For this review, take the finished solid that the model builds, in its own axes (mm). A direction names the side the tool comes from. Round coordinates to 2 decimals unless told otherwise and drop trailing zeros. Loops run counter-clockwise (first coordinate to the right, second up) from the corner with the lowest first, then second, coordinate; pieces in that order, holes last.
1. Clearance check with flat-ended pins moving along their axes: pin 1 Ø3 at (x, z) = (-18.25, 14) entering from -Y; pin 2 Ø1.2 at (x, y) = (-29.25, -8) entering from +Z. State where each tip first meets the part, or that it passes through.
2. Consider section C-C on z = 3. State the section outline as (x, y) points, then the cut area to 3 significant figures.
3. To check wall thickness, follow line 1 along Y through (x, z) = (29.25, -8); line 2 along Y through (x, z) = (-30, 1.5); line 3 along X through (y, z) = (-31.5, 7.5). State the ranges of each line that lie inside material, in increasing order.
4. Consider section D-D on z = 14. State the section outline as (x, y) points, then the cut area to 3 significant figures.
5. Consider section B-B on x = 23.75. State the section outline as (y, z) points.
6. Consider section A-A on y = -32. State the section outline as (x, z) points, then the cut area to 3 significant figures.
7. Draft analysis for pull direction Z (two halves, no side actions). For faces 1 (the cylindrical face through (-18.467, -19.72, -14.976)), 2 (the flat face through (-37.25, -20, 3)), 3 (the flat face through (-23, -20, -16.25)), 4 (the cylindrical face through (-18.248, -19.72, -0.281)), state which applies: released by +Z, released by -Z, zero draft, split by the parting line, or undercut.
8. Tool access review of faces 5 (the cylindrical face through (30.204, -7.7, 3.016)), 6 (the flat face through (0, -20, 16.25)): name each direction out of +Z, -Z, +X, -X, +Y, -Y from which nothing blocks a thin tool from reaching the whole face with its end or side.
from build123d import *

# Parameters (mm, degrees)
F0_R     = 1
F1_DEPTH = 40
F2_R     = 1
F3_DEPTH = 46.1


with BuildPart() as f1:
    # F0 (on Front) → F1 (new body)
    with BuildSketch(Plane.XZ):
        with BuildLine():
            Line((-8.306624, 16.25), (-37.25, 16.25))
            Line((-37.25, 16.25), (-37.25, -16.25))
            Line((-37.25, -16.25), (-8.306624, -16.25))
            ThreePointArc((-8.306624, -16.25), (-18.25, 0), (-8.306624, 16.25))
        make_face()
        with Locations((-18.25, -14)):
            Circle(F0_R, mode=Mode.SUBTRACT)
        with Locations((-18.25, 14)):
            Circle(F0_R, mode=Mode.SUBTRACT)
        with BuildLine():
            Line((37.25, 21.75), (-37.25, 21.75))
            Line((-37.25, 21.75), (-37.25, 16.25))
            Line((-37.25, 16.25), (-8.306624, 16.25))
            ThreePointArc((-8.306624, 16.25), (0, 18.25), (8.306624, 16.25))
            Line((8.306624, 16.25), (37.25, 16.25))
            Line((37.25, 16.25), (37.25, 21.75))
        make_face()
        with BuildLine():
            Line((37.25, -16.25), (37.25, 16.25))
            Line((37.25, 16.25), (8.306624, 16.25))
            ThreePointArc((8.306624, 16.25), (15.566926, 9.525403), (18.25, 0))
            ThreePointArc((18.25, 0), (15.566926, -9.525403), (8.306624, -16.25))
            Line((8.306624, -16.25), (37.25, -16.25))
        make_face()
        with Locations((23.75, 0)):
            Circle(F0_R, mode=Mode.SUBTRACT)
        with BuildLine():
            ThreePointArc((8.306624, 16.25), (0, 18.25), (-8.306624, 16.25))
            Line((-8.306624, 16.25), (8.306624, 16.25))
        make_face()
    extrude(amount=F1_DEPTH)

    # F2 (on face) → F3 (cut)
    with BuildSketch(Plane.XY.offset(21.75)):
        with Locations((-29.25, -8)):
            Circle(F2_R)
        with Locations((-29.25, -32)):
            Circle(F2_R)
        with Locations((29.25, -32)):
            Circle(F2_R)
        with Locations((29.25, -8)):
            Circle(F2_R)
    extrude(amount=-F3_DEPTH, mode=Mode.SUBTRACT)


solid = f1.part
Resolved:
1. pin 1: stops at y = -40
1. pin 2: passes through
2. outline: (-37.25, -40) - (-18, -40) - (-18, 0) - (-37.25, 0) - close; (18, -40) - (37.25, -40) - (37.25, 0) - (18, 0) - close; hole circle Ø2 at (-29.25, -32); hole circle Ø2 at (-29.25, -8); hole circle Ø2 at (29.25, -32); hole circle Ø2 at (29.25, -8)
2. area: 1,530 mm2
3. line 1: y = -40 to -33, -31 to -9, -7 to 0
3. line 2: y = -40 to -32.66, -31.34 to -8.66, -7.34 to 0
3. line 3: x = -37.25 to -30.12, -28.38 to -16.64, 16.64 to 28.38, 30.12 to 37.25
4. outline: (-37.25, -40) - (-19.25, -40) - (-19.25, 0) - (-37.25, 0) - close; (-17.25, -40) - (-11.71, -40) - (-11.71, 0) - (-17.25, 0) - close; (11.71, -40) - (37.25, -40) - (37.25, 0) - (11.71, 0) - close; hole circle Ø2 at (-29.25, -32); hole circle Ø2 at (-29.25, -8); hole circle Ø2 at (29.25, -32); hole circle Ø2 at (29.25, -8)
4. area: 1,950 mm2
5. outline: (-40, -16.25) - (0, -16.25) - (0, -1) - (-40, -1) - close; (-40, 1) - (0, 1) - (0, 21.75) - (-40, 21.75) - close
6. outline: (-37.25, -16.25) - (-30.25, -16.25) - (-30.25, 21.75) - (-37.25, 21.75) - close; (-28.25, -16.25) - (-8.31, -16.25) arc R18.25 cw to (-8.31, 16.25) - (8.31, 16.25) arc R18.25 cw to (18.25, 0) arc R18.25 cw to (8.31, -16.25) - (28.25, -16.25) - (28.25, 21.75) - (-28.25, 21.75) - close; (30.25, -16.25) - (37.25, -16.25) - (37.25, 21.75) - (30.25, 21.75) - close; hole circle Ø2 at (-18.25, -14); hole circle Ø2 at (-18.25, 14); hole circle Ø2 at (23.75, 0)
6. area: 1,670 mm2
7. face 1: undercut
7. face 2: zero draft
7. face 3: released by -Z
7. face 4: undercut
8. face 5: +Z, -Z
8. face 6: -Z, +Y, -Y
